```python
from build123d import *

# Parameters (mm, degrees)
F0_W     = 33.02
F0_H     = 127
F1_ANGLE = 240
F2_W     = 20.32
F2_H     = 114.3


with BuildPart() as f1:
    # F0 (on Front) → F1 (revolve, symmetric)
    with BuildSketch(Plane.XZ) as f1_sk:
        with Locations((-16.722997, -11.941442)):
            Rectangle(F0_W, F0_H)
    revolve(axis=Axis((-0.212997, 0, -11.941442), (0, 0, -1)), revolution_arc=F1_ANGLE / 2)
    revolve(f1_sk.sketch, axis=Axis((-0.212997, 0, -11.941442), (0, 0, 1)), revolution_arc=F1_ANGLE / 2)

    # F2 (on Front) → F3 (revolve, cut)
    with BuildSketch(Plane.XZ):
        with Locations((-10.534671, -10.423937)):
            Rectangle(F2_W, F2_H)
    revolve(axis=Axis((-0.374671, 0, -10.423937), (0, 0, -1)), mode=Mode.SUBTRACT)


solid = f1.part
```
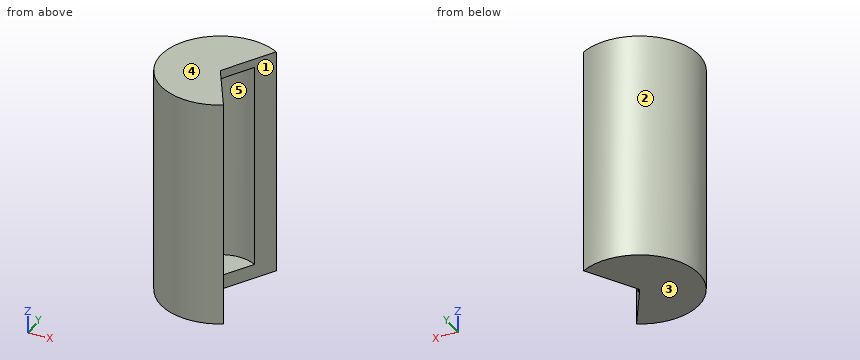
Check sheet for the modelled part. Datum: model origin and axes. Units: mm. Face numbers are marked on the shaded views. A direction names the side the tool comes from. Give positions to 0.01 mm unless a question says otherwise; leave off trailing zeros. Order: outer loops, then holes, each group sorted by start corner. A loop starts at its lowest first (then second) coordinate and runs counter-clockwise, first axis right, second up. Notation, with made-up numbers: M -15.75,54.25 L 39.25,54.25 A14 cw 39.25,75.25 Z; hole C 31,-30 d9. An arc over 180 degrees is marked long. Answer in a Markdown table with one row per item. Add a question column.
Q1. Gauge pin test, flat ends, axial feed: pin 1 Ø3 at (y, z) = (23.5, -28) entering from +X; pin 2 Ø12 at (x, z) = (-27.5, -8) entering from +Y; pin 3 Ø4 at (x, z) = (-15, -62) entering from -Y. Record the tip position at first contact, or that the pin passes through.
Q2. Access from +Z, -Z, +X, -X, +Y, -Y to the whole of each face (thin tool, end or side, straight path). Record for the marked faces 4 and 5.
Q3. Sectioned sample at B-B, the plane y = 11. Record the boundary of the cut face in (x, z).
Q4. Sectioned sample at C-C, the plane x = -4. Record the boundary of the cut face in (y, z), and give its area (3 significant figures).
Q5. Sectioned sample at A-A, the plane x = 3.5. Record the boundary of the cut face in (y, z), and give its area (3 significant figures).
Q6. Sectioned sample at D-D, the plane y = -14. Record the boundary of the cut face in (x, z).
Q7. Release check for a two-part mould opening along Y. For the marked faces 1, 2 and 3 record: released by +Y, released by -Y, zero draft, split by the parting line, or undercut.
Q8. Thickness scan on L1, parallel to Z at x = -4.5, y = 16.5; L2, parallel to Y at x = -0.5, z = 14.5; L3, parallel to X at y = 0, z = -30. Record the ranges inside material, lowest first.
Verdict:
| question | item | result |
|---|---|---|
| 1 | pin 1 | x = 14.22 |
| 1 | pin 2 | y = 25.24 |
| 1 | pin 3 | y = -30.44 |
| 2 | face 4 | +Z, +X, -X, +Y, -Y |
| 2 | face 5 | none |
| 3 | outline | M -31.35,-75.44 L 6.14,-75.44 L 6.14,-67.57 L -17.46,-67.57 L -17.46,46.73 L 6.14,46.73 L 6.14,51.56 L -31.35,51.56 Z |
| 4 | outline | M -32.8,-75.44 L 32.8,-75.44 L 32.8,51.56 L -32.8,51.56 Z; hole M -19.99,-67.57 L 19.99,-67.57 L 19.99,46.73 L -19.99,46.73 Z |
| 4 | area | 3,760 mm² |
| 5 | outline | M -32.81,-75.44 L -6.43,-75.44 L -6.43,-67.57 L -19.95,-67.57 L -19.95,46.73 L -6.43,46.73 L -6.43,51.56 L -32.81,51.56 Z; M 6.43,-75.44 L 32.81,-75.44 L 32.81,51.56 L 6.43,51.56 L 6.43,46.73 L 19.95,46.73 L 19.95,-67.57 L 6.43,-67.57 Z |
| 5 | area | 3,610 mm² |
| 6 | outline | M -30.12,-75.44 L 7.87,-75.44 L 7.87,-67.57 L -15.1,-67.57 L -15.1,46.73 L 7.87,46.73 L 7.87,51.56 L -30.12,51.56 Z |
| 7 | face 1 | undercut |
| 7 | face 2 | split by the parting line |
| 7 | face 3 | zero draft |
| 8 | L1 | -75.44 to -67.57, 46.73 to 51.56 |
| 8 | L2 | -33.02 to -20.32, 20.32 to 33.02 |
| 8 | L3 | -33.23 to -20.69 |
